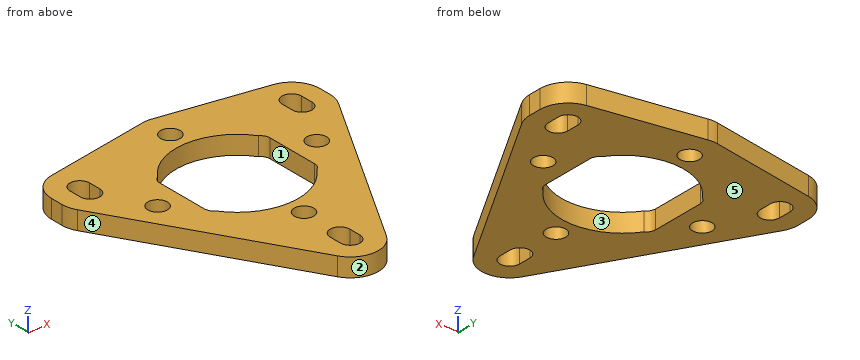
Autodesk Inventor part; units mm, degrees
ref_plane "YZ Plane" through (0, 0, 0) normal (1, 0, 0) x (0, 1, 0)
ref_plane "XZ Plane" through (0, 0, 0) normal (0, 1, 0) x (-1, 0, 0)
ref_plane "XY Plane" through (0, 0, 0) normal (0, 0, 1) x (1, 0, 0)
sketch "スケッチ1" plane through (0, 0, 0) normal (0, 0, 1) x (1, 0, 0)
  line L0 (9, -4.3589) -> (9, 4.3589)
  line L1 (-9, 4.3589) -> (-9, -4.3589)
  arc A0 (8.2425, 5.6622) -> (-8.2425, 5.6622) centre (0, 0) ccw
  arc A1 (-8.2425, 5.6622) -> (-9, 4.3589) centre (-7.5, 4.3589) ccw
  arc A2 (9, 4.3589) -> (8.2425, 5.6622) centre (7.5, 4.3589) ccw
  arc A3 (8.2425, -5.6622) -> (9, -4.3589) centre (7.5, -4.3589) ccw
  arc A4 (-9, -4.3589) -> (-8.2425, -5.6622) centre (-7.5, -4.3589) ccw
  arc A5 (-8.2425, -5.6622) -> (8.2425, -5.6622) centre (0, 0) ccw
  line L2 (-9, 0) -> (9, 0) construction
  line L3 (-13, 0) -> (-13, 0) construction
  line L4 (-14.6, 0) -> (-14.6, 0)
  line L5 (-11.4, 0) -> (-11.4, 0)
  arc A6 (-11.4, 0) -> (-14.6, 0) centre (-13, 0) ccw
  arc A7 (-14.6, 0) -> (-11.4, 0) centre (-13, 0) ccw
  line L6 (25, -30) -> (-25, -30)
  line L7 (-25, -30) -> (-25, 30)
  line L8 (-25, 30) -> (25, 30)
  line L9 (25, 30) -> (25, -30)
  line L10 (25, -30) -> (-25, 30) construction
  line L11 (-25, -30) -> (25, 30) construction
  line L12 (13, 0) -> (13, 0) construction
  line L13 (11.4, 0) -> (11.4, 0)
  line L14 (14.6, 0) -> (14.6, 0)
  arc A8 (14.6, 0) -> (11.4, 0) centre (13, 0) ccw
  arc A9 (11.4, 0) -> (14.6, 0) centre (13, 0) ccw
  line L15 (0, 13) -> (0, 13) construction
  line L16 (-1.6, 13) -> (-1.6, 13)
  line L17 (1.6, 13) -> (1.6, 13)
  arc A10 (1.6, 13) -> (-1.6, 13) centre (0, 13) ccw
  arc A11 (-1.6, 13) -> (1.6, 13) centre (0, 13) ccw
  line L18 (0, -13) -> (0, -13) construction
  line L19 (1.6, -13) -> (1.6, -13)
  line L20 (-1.6, -13) -> (-1.6, -13)
  arc A12 (-1.6, -13) -> (1.6, -13) centre (0, -13) ccw
  arc A13 (1.6, -13) -> (-1.6, -13) centre (0, -13) ccw
  point P0 (0, 0)
  point P1 (0, 13)
  point P2 (0, -13)
  dimension "d2" = 18
  dimension "d3" = 3
  dimension "d5" = 10
  dimension "d6" = 0
  dimension "d7" = 10
  dimension "d8" = 3.2
  dimension "d9" = 13
  dimension "d10" = 0
  dimension "d11" = 50
  dimension "d12" = 60
  dimension "d22" = 13
  dimension "d23" = 13
  dimension "d24" = 13
extrude "押し出し1" add sketch "スケッチ1" along normal blind 3
sketch "スケッチ3" plane through (0, 0, 3) normal (0, 0, 1) x (1, 0, 0)
  line L0 (0, -22) -> (0, -20) construction
  line L1 (1.6, -22) -> (1.6, -20)
  line L2 (-1.6, -20) -> (-1.6, -22)
  arc A0 (-1.6, -22) -> (1.6, -22) centre (0, -22) ccw
  arc A1 (1.6, -20) -> (-1.6, -20) centre (0, -20) ccw
  line L3 (-17.3205, 10) -> (-17.3205, 8) construction
  line L4 (-18.9205, 10) -> (-18.9205, 8)
  line L5 (-15.7205, 8) -> (-15.7205, 10)
  arc A2 (-15.7205, 10) -> (-18.9205, 10) centre (-17.3205, 10) ccw
  arc A3 (-18.9205, 8) -> (-15.7205, 8) centre (-17.3205, 8) ccw
  line L6 (17.3205, 10) -> (17.3205, 8) construction
  line L7 (15.7205, 10) -> (15.7205, 8)
  line L8 (18.9205, 8) -> (18.9205, 10)
  arc A4 (18.9205, 10) -> (15.7205, 10) centre (17.3205, 10) ccw
  arc A5 (15.7205, 8) -> (18.9205, 8) centre (17.3205, 8) ccw
  circle A6 centre (0, 0) radius 20 construction
  point P0 (0, -21)
  point P1 (-17.3205, 9)
  point P2 (17.3205, 9)
  dimension "d26" = 2
  dimension "d27" = 1.6
  dimension "d28" = 20
  dimension "d29" = 120
extrude "押し出し4" cut sketch "スケッチ3" against normal blind 3
sketch "スケッチ4" plane through (0, 0, 3) normal (0, 0, 1) x (1, 0, 0)
  arc A0 (-18.9205, 8) -> (-15.7205, 8) centre (-17.3205, 8) ccw
  line L0 (-18.9205, 8) -> (-18.9205, 10)
  arc A1 (-15.7205, 10) -> (-18.9205, 10) centre (-17.3205, 10) ccw
  line L1 (-15.7205, 10) -> (-15.7205, 8)
  arc A2 (1.6, -20) -> (-1.6, -20) centre (0, -20) ccw
  line L2 (1.6, -20) -> (1.6, -22)
  arc A3 (-1.6, -22) -> (1.6, -22) centre (0, -22) ccw
  line L3 (-1.6, -22) -> (-1.6, -20)
  arc A4 (15.7205, 8) -> (18.9205, 8) centre (17.3205, 8) ccw
  line L4 (15.7205, 8) -> (15.7205, 10)
  arc A5 (18.9205, 10) -> (15.7205, 10) centre (17.3205, 10) ccw
  line L5 (18.9205, 10) -> (18.9205, 8)
  arc A6 (8.2425, -5.6622) -> (9, -4.3589) centre (7.5, -4.3589) ccw
  arc A7 (-8.2425, -5.6622) -> (8.2425, -5.6622) centre (0, 0) ccw
  arc A8 (-9, -4.3589) -> (-8.2425, -5.6622) centre (-7.5, -4.3589) ccw
  line L6 (-9, -4.3589) -> (-9, 4.3589)
  arc A9 (-8.2425, 5.6622) -> (-9, 4.3589) centre (-7.5, 4.3589) ccw
  arc A10 (8.2425, 5.6622) -> (-8.2425, 5.6622) centre (0, 0) ccw
  arc A11 (9, 4.3589) -> (8.2425, 5.6622) centre (7.5, 4.3589) ccw
  line L7 (9, 4.3589) -> (9, -4.3589)
  circle A12 centre (0, -13) radius 1.6
  circle A13 centre (0, 13) radius 1.6
  circle A14 centre (13, 0) radius 1.6
  circle A15 centre (-13, 0) radius 1.6
  line L8 (-25, -30) -> (25, -30)
  line L9 (25, -30) -> (25, 30)
  line L10 (25, 30) -> (-25, 30)
  line L11 (-25, 30) -> (-25, -30)
  arc A16 (-21.9205, 8) -> (-12.7205, 8) centre (-17.3205, 8) ccw
  line L12 (-21.9205, 8) -> (-21.9205, 10)
  arc A17 (-12.7205, 10) -> (-21.9205, 10) centre (-17.3205, 10) ccw
  line L13 (-12.7205, 10) -> (-12.7205, 8)
  line L14 (12.7205, 10) -> (12.7205, 8)
  arc A18 (12.7205, 8) -> (21.9205, 8) centre (17.3205, 8) ccw
  line L15 (21.9205, 8) -> (21.9205, 10)
  arc A19 (21.9205, 10) -> (12.7205, 10) centre (17.3205, 10) ccw
  circle A20 centre (0, 13) radius 4.6
  arc A21 (4.6, -20) -> (-4.6, -20) centre (0, -20) ccw
  line L16 (4.6, -20) -> (4.6, -22)
  arc A22 (-4.6, -22) -> (4.6, -22) centre (0, -22) ccw
  line L17 (-4.6, -22) -> (-4.6, -20)
  line L18 (-3.9837, -24.3) -> (-21.3042, 5.7)
  line L19 (3.9837, -24.3) -> (21.3042, 5.7)
  line L20 (0.7851, 17.5325) -> (18.1056, 14.5325)
  line L21 (-0.7851, 17.5325) -> (-18.1056, 14.5325)
  dimension "d32" = 3
  dimension "d33" = 3
  dimension "d34" = 3
  dimension "d35" = 3
extrude "押し出し5" cut sketch "スケッチ4" against normal blind 3 contours L0 A1 L1 A0 | L2 A3 L3 A2 | L4 A5 L5 A4 | A7 A8 L6 A9 A10 A20 A11 L7 A6 | A6 L7 A11 A10 A20 L20 A19 L14 A18 L19 A22 L16 A21 L17 L18 A16 L13 A17 L21 A9 L6 A8 A7 | A20 A10 | A10 A20 | A17 L13 A16 L12 | A19 L15 A18 L14 | A22 L17 A21 L16 | A12 | A13 | A14 | A15 keep common part
equation "\"d22\" = d9"
equation "\"d23\" = d9"
properties part number "RS555-71Mount"
The model under review builds one solid part; all positions refer to its coordinate system, in mm. Face numbers are marked on the shaded views. A direction names the side the tool comes from. Give positions to 0.01 mm unless a question says otherwise; leave off trailing zeros. Order: outer loops, then holes, each group sorted by start corner. A loop starts at its lowest first (then second) coordinate and runs counter-clockwise, first axis right, second up. Notation, with made-up numbers: M -6,-31.5 L 50,-31.5 A25 ccw 50,-11.5 Z; hole C -10.75,6.25 d3. An arc over 180 degrees is marked long. Answer in a Markdown table with one row per item. Add a question column.
1. Mouldability with a two-part tool opening along X and no side actions: class the marked faces 3, 4 and 5 as released by +X, released by -X, zero draft, split by the parting line, or undercut.
2. Add section D-D on y = 0. State the section outline as (x, z) points.
3. Add section B-B on y = -13. State the section outline as (x, z) points, plus the area to 3 significant figures.
4. Add section C-C on x = 14. State the section outline as (y, z) points.
5. For pin 1 Ø1 at (y, z) = (-21, 2) entering from -X; pin 2 Ø1 at (x, z) = (-6, 1.5) entering from +Y; pin 3 Ø1 at (y, z) = (-21, 1.5) entering from +X, all flat-tipped, find the tip position at first contact; note any pin that passes through.
6. Machinability: for the marked faces 1 and 2, which of the approach directions +Z, -Z, +X, -X, +Y, -Y give a long, thin tool a straight path to every point of the face, cutting with its end or side? Answer none if there is none.
7. To check wall thickness, follow line 1 along X through (y, z) = (0, 1.05); line 2 along Y through (x, z) = (-17.5, 2.35); line 3 along X through (y, z) = (13, 1.7). State the ranges of each line that lie inside material, in increasing order.
8. Add section A-A on x = 0. State the section outline as (y, z) points, plus the area to 3 significant figures.
The answers:
| question | item | result |
|---|---|---|
| 1 | face 3 | undercut |
| 1 | face 4 | released by -X |
| 1 | face 5 | zero draft |
| 2 | outline | M -18.01,0 L -14.6,0 L -14.6,3 L -18.01,3 Z; M -11.4,0 L -9,0 L -9,3 L -11.4,3 Z; M 9,0 L 11.4,0 L 11.4,3 L 9,3 Z; M 14.6,0 L 18.01,0 L 18.01,3 L 14.6,3 Z |
| 3 | outline | M -10.51,0 L -1.6,0 L -1.6,3 L -10.51,3 Z; M 1.6,0 L 10.51,0 L 10.51,3 L 1.6,3 Z |
| 3 | area | 53.4 mm2 |
| 4 | outline | M -6.95,0 L -1.25,0 L -1.25,3 L -6.95,3 Z; M 1.25,0 L 15.24,0 L 15.24,3 L 1.25,3 Z |
| 5 | pin 1 | x = -6.18 |
| 5 | pin 2 | y = 16.72 |
| 5 | pin 3 | x = 6.18 |
| 6 | face 1 | +Z, -Z |
| 6 | face 2 | +Z, -Z, -Y |
| 7 | line 1 | -18.01 to -14.6, -11.4 to -9, 9 to 11.4, 14.6 to 18.01 |
| 7 | line 2 | -0.89 to 6.41, 11.59 to 14.64 |
| 7 | line 3 | -20.81 to -1.6, 1.6 to 20.81 |
| 8 | outline | M -26.6,0 L -23.6,0 L -23.6,3 L -26.6,3 Z; M -18.4,0 L -14.6,0 L -14.6,3 L -18.4,3 Z; M -11.4,0 L -10,0 L -10,3 L -11.4,3 Z; M 10,0 L 11.4,0 L 11.4,3 L 10,3 Z; M 14.6,0 L 17.6,0 L 17.6,3 L 14.6,3 Z |
| 8 | area | 37.8 mm2 |
